Part print with two shaded views. Sizes in mm from the minimum x, y, z corner. A direction names the side the tool comes from. Round coordinates to 2 decimals unless told otherwise and drop trailing zeros. Write each loop counter-clockwise with the first axis right and the second up, starting at its lowest first coordinate (ties: lowest second). Pieces come first, ordered by that corner, then holes.
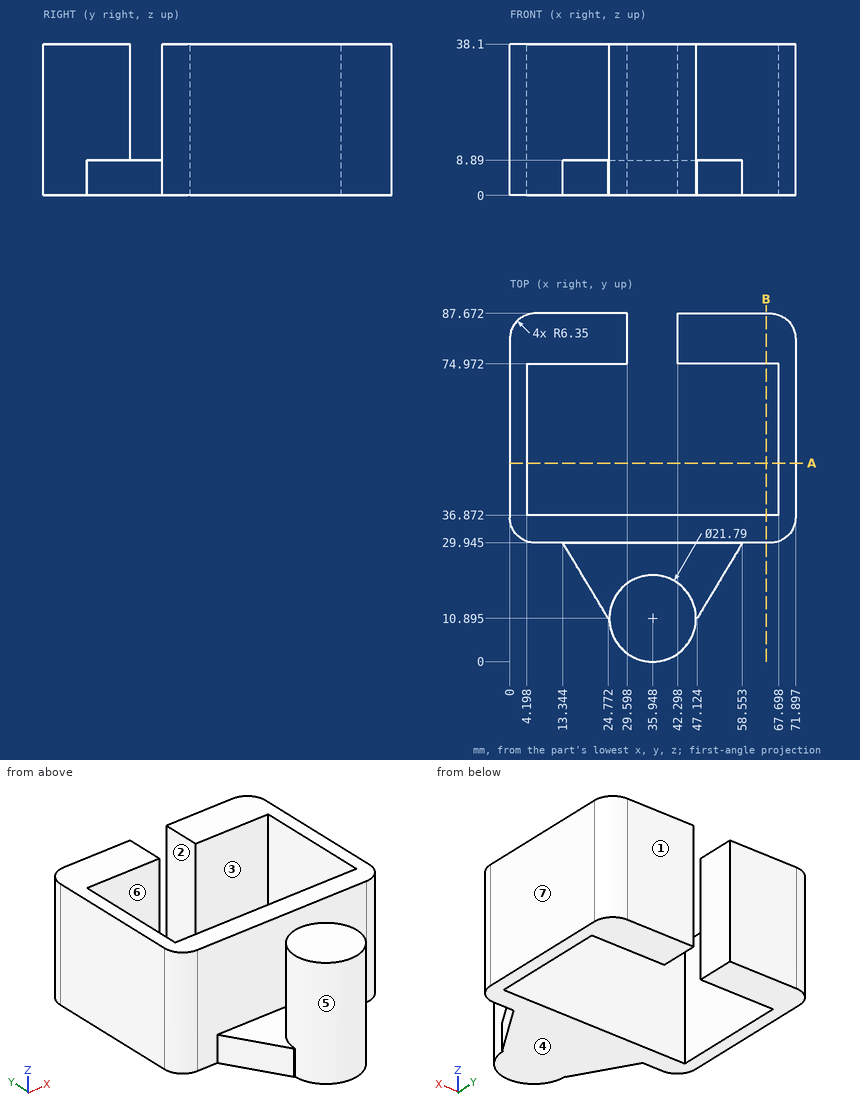
Q1. Mould opens along X. For the marked faces 4, 5, 6 and 7 say: +X half, -X half, draft (parallel to the pull), parting line (faces both ways), or undercut.
Values follow:
face 4: draft
face 5: parting line
face 6: undercut
face 7: +X half
Q2. Cut at A-A on y = 50. Write the cut outline in (x, z).
Values follow:
outline: (0, 0) - (4.2, 0) - (4.2, 38.1) - (0, 38.1) - close; (67.7, 0) - (71.9, 0) - (71.9, 38.1) - (67.7, 38.1) - close
Q3. Drop flat-ended pins along their axis: pin 1 (5 mm diameter, centred on y = 10.5, z = 22, fed in from -X); pin 2 (7.5 mm diameter, centred on x = 19, z = 16.5, fed in from -Y) (3 decimals); pin 3 (8 mm diameter, centred on y = 17.5, z = 25.5, fed in from -X). Give the stop position or say it passes through.
Values follow:
pin 1: stops at x = 25.05
pin 2: stops at y = 29.945
pin 3: stops at x = 25.37
Q4. Wall check: L1, parallel to X at y = 71.5, z = 22; L2, parallel to Y at x = 56, z = 34.5 (1 decimal); L3, parallel to X at y = 80, z = 2.5. Give the ranges that are in metal, low to high.
Values follow:
L1: x = 0 to 4.2, 67.7 to 71.9
L2: y = 29.9 to 36.9, 75 to 87.7
L3: x = 0 to 29.6, 42.3 to 71.9
Q5. Cut at B-B on x = 64.5. Write the cut outline in (y, z) (1 decimal).
Values follow:
outline: (29.9, 0) - (36.9, 0) - (36.9, 38.1) - (29.9, 38.1) - close; (75, 0) - (87.7, 0) - (87.7, 38.1) - (75, 38.1) - close
Q6. Which spindle directions (+Z, -Z, +X, -X, +Y, -Y) get a long thin tool onto all of the face, cutting with end or side? Do the marked faces 1, 2 and 3. Say none if no direction does.
Values follow:
face 1: +Z, -Z, +X, -X, +Y
face 2: +Z, -Z, +Y
face 3: +Z, -Z
